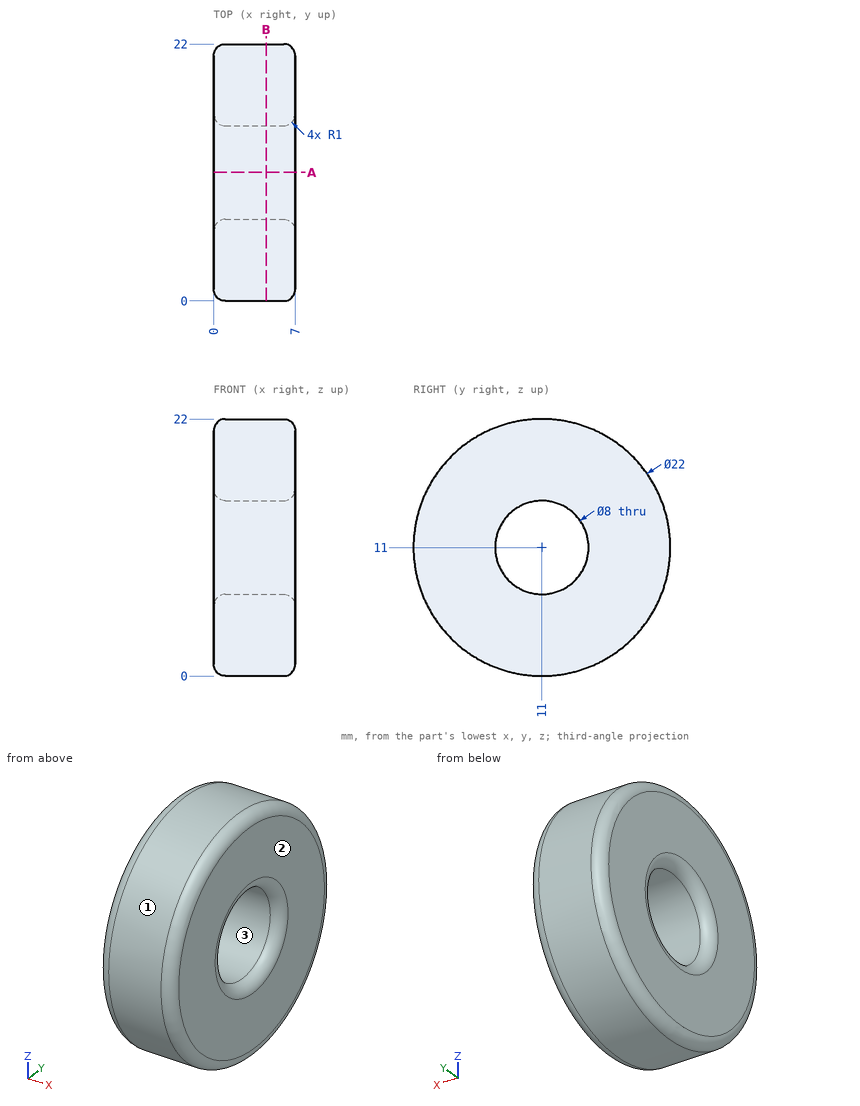
Could you check a few things on this drawing? It's one solid part, dimensions in mm from its lowest x, y, z. Coordinates: 2 decimals unless noted, no trailing zeros. Loops run counter-clockwise (first coordinate to the right, second up) from the corner with the lowest first, then second, coordinate; pieces in that order, holes last. Notation, with made-up numbers: (33.5, -16.75) - (91.5, -16.75) arc R18 cw to (91.5, 18.25) - close; hole circle Ø3 at (-12.5, -18). An arc over 180 degrees is marked (long way). Return JSON: item names as keys, results as strings. Group by question number.
Item 1: I need wall thicknesses on line 1 (Z direction, x = 3.45, y = 11); line 2 (Z direction, x = 0.5, y = 15.25); line 3 (Z direction, x = 2.25, y = 12.25). Which ranges of each line are inside material? Lowest first, please. Write a range as from..to.
Item 2: Will these pins go through, and if not, where does the flat tip stop? P1, Ø2, axis at x = 0.5, z = 15.5, coming from the -Y side; P2, Ø1.5, axis at x = 1, z = 14, coming from the +Y side; P3, Ø1.5, axis at x = 5.5, z = 3.5, coming from the +Y side.
Item 3: We'd pull the mould along Z, two halves only. Please class the marked faces 1, 2 and 3: +Z half, -Z half, draft (parallel to the pull), parting line (faces both ways), or undercut.
Item 4: If we section it at A-A on y = 11: Write out the boundary of the cut face in (x, z), and give its area (3 significant figures).
Item 5: If we section it at B-B on x = 4.5: Write out the boundary of the cut face in (y, z), and give its area (3 significant figures).
Calculated:
{
 "1": {"line 1": "z = 0..7, 15..22", "line 2": "z = 1..21", "line 3": "z = 0.07..7.2, 14.8..21.93"},
 "2": {"P1": "stops at y = 0.6", "P2": "stops at y = 21.77", "P3": "stops at y = 19.69"},
 "3": {"face 1": "parting line", "face 2": "draft", "face 3": "undercut"},
 "4": {"outline": "(0, 1) arc R1 ccw to (1, 0) - (6, 0) arc R1 ccw to (7, 1) - (7, 6) arc R1 ccw to (6, 7) - (1, 7) arc R1 ccw to (0, 6) - close; (0, 16) arc R1 ccw to (1, 15) - (6, 15) arc R1 ccw to (7, 16) - (7, 21) arc R1 ccw to (6, 22) - (1, 22) arc R1 ccw to (0, 21) - close", "area": "96.3 mm^2"},
 "5": {"outline": "circle Ø22 at (11, 11); hole circle Ø8 at (11, 11)", "area": "330 mm^2"}
}
